from build123d import *

# Parameters (mm, degrees)
SKETCH1_W           = 25.4
SKETCH1_H           = 127
BOSS_EXTRUDE1_DEPTH = 6.35
SKETCH2_R           = 1.190625
CUT_EXTRUDE1_DEPTH  = 6.35
FILLET1_R           = 6.35
SKETCH3_R           = 4.7625
CUT_EXTRUDE2_DEPTH  = 6.35
FILLET2_R           = 6.35
SKETCH4_R           = 11.1125
CUT_EXTRUDE3_DEPTH  = 1.5875
SKETCH5_R           = 1.5875
CUT_EXTRUDE4_DEPTH  = 6.35


with BuildPart() as part:
    # Sketch1 → Boss-Extrude1 (new body)
    with BuildSketch(Plane.XY):
        with Locations((12.7, 63.5)):
            Rectangle(SKETCH1_W, SKETCH1_H)
    extrude(amount=BOSS_EXTRUDE1_DEPTH)

    # Sketch2 → Cut-Extrude1 (cut)
    with BuildSketch(Plane.XY.offset(6.35)):
        with Locations((5.7, 4.7625)):
            Circle(SKETCH2_R)
        with Locations((19.7, 4.7625)):
            Circle(SKETCH2_R)
        with Locations((12.7, 11.7625)):
            Circle(SKETCH2_R)
    extrude(amount=-CUT_EXTRUDE1_DEPTH, mode=Mode.SUBTRACT)

    # Fillet1
    fillet1_edges = [part.edges().sort_by_distance(p)[0] for p in [
        (25.4, 0, 3.175),
        (0, 0, 3.175),
    ]]
    fillet(fillet1_edges, radius=FILLET1_R)

    # Sketch3 → Cut-Extrude2 (cut)
    with BuildSketch(Plane.XY.offset(6.35)):
        with Locations((12.7, 110.499906)):
            Circle(SKETCH3_R)
    extrude(amount=-CUT_EXTRUDE2_DEPTH, mode=Mode.SUBTRACT)

    # Fillet2
    fillet2_edges = [part.edges().sort_by_distance(p)[0] for p in [
        (0, 127, 3.175),
        (25.4, 127, 3.175),
    ]]
    fillet(fillet2_edges, radius=FILLET2_R)

    # Sketch4 → Cut-Extrude3 (cut)
    with BuildSketch(Plane.XY.offset(6.35)):
        with Locations((12.7, 110.499906)):
            Circle(SKETCH4_R)
    extrude(amount=-CUT_EXTRUDE3_DEPTH, mode=Mode.SUBTRACT)

    # Sketch5 → Cut-Extrude4 (cut)
    with BuildSketch(Plane.XY.offset(6.35)):
        with Locations((17.7, 124)):
            Circle(SKETCH5_R)
        with Locations((7.7, 124)):
            Circle(SKETCH5_R)
        with Locations((17.7, 76)):
            Circle(SKETCH5_R)
        with Locations((7.7, 76)):
            Circle(SKETCH5_R)
    extrude(amount=-CUT_EXTRUDE4_DEPTH, mode=Mode.SUBTRACT)


solid = part.part
Read the model definition and answer for the solid it produces. Units are mm, in the model's axes. A direction names the side the tool comes from. Coordinates: 2 decimals unless noted, no trailing zeros. Loops run counter-clockwise (first coordinate to the right, second up) from the corner with the lowest first, then second, coordinate; pieces in that order, holes last.
Q1. The part is cut by section B-B on x = 12.7. Write down the section's boundary in (y, z), and give its area (3 significant figures).
Q2. Which of the six approach directions +Z, -Z, +X, -X, +Y, -Y give full straight-line access (tool end or side, diameter ignored) to faces 1 (the face through (17, 108, 4.762)), 2 (the face through (23.49, 125.19, 3.22))?
Q3. The part is cut by section A-A on y = 76. Write down the section's boundary in (x, z).
Q4. The part is cut by section D-D on y = 109. Write down the section's boundary in (x, z).
Q5. This flat-tipped pin is pushed along its axis until it touches: pin 1 Ø1.9 at (x, y) = (17.7, 124) entering from -Z. Where does it stop, or does it pass through?
Q6. Consider probe 1 along X at (y, z) = (76, 5.25); probe 2 along Y at (x, z) = (7.7, 3); probe 3 along Y at (x, z) = (12.7, 5.7). Determine where each line is inside the solid, lowest interval first.
Q7. The part is cut by section C-C on z = 3.25. Give the number of separate pieces and of enclosed holes in the cut face, and give its area (3 significant figures).
Results below:
1. outline: (0, 0) - (10.57, 0) - (10.57, 6.35) - (0, 6.35) - close; (12.95, 0) - (105.74, 0) - (105.74, 4.76) - (99.39, 4.76) - (99.39, 6.35) - (12.95, 6.35) - close; (115.26, 0) - (127, 0) - (127, 6.35) - (121.61, 6.35) - (121.61, 4.76) - (115.26, 4.76) - close
1. area: 711 mm2
2. face 1: +Z
2. face 2: +Z, -Z, +X, +Y
3. outline: (0, 0) - (6.11, 0) - (6.11, 6.35) - (0, 6.35) - close; (9.29, 0) - (16.11, 0) - (16.11, 6.35) - (9.29, 6.35) - close; (19.29, 0) - (25.4, 0) - (25.4, 6.35) - (19.29, 6.35) - close
4. outline: (0, 0) - (8.18, 0) - (8.18, 4.76) - (1.69, 4.76) - (1.69, 6.35) - (0, 6.35) - close; (17.22, 0) - (25.4, 0) - (25.4, 6.35) - (23.71, 6.35) - (23.71, 4.76) - (17.22, 4.76) - close
5. pin 1: passes through
6. probe 1: x = 0 to 6.11, 9.29 to 16.11, 19.29 to 25.4
6. probe 2: y = 0 to 74.41, 77.59 to 122.41, 125.59 to 127
6. probe 3: y = 0 to 10.57, 12.95 to 99.39, 121.61 to 127
7. separate pieces: 1
7. enclosed holes: 8
7. area: 3,070 mm2
